Work out the finished part from the listing and answer in its coordinate system (mm). Round coordinates to 2 decimals unless told otherwise and drop trailing zeros. Order: outer loops, then holes, each group sorted by start corner. A loop starts at its lowest first (then second) coordinate and runs counter-clockwise, first axis right, second up. Notation, with made-up numbers: M 15,63 L 69,63 A14 ccw 69,79 Z; hole C 66,21 d8. An arc over 180 degrees is marked long. Answer as a JSON object with one key per item and string values. Group by question number.
Autodesk Inventor part; units mm, degrees
ref_plane "YZ Plane" through (0, 0, 0) normal (1, 0, 0) x (0, 1, 0)
ref_plane "XZ Plane" through (0, 0, 0) normal (0, 1, 0) x (-1, 0, 0)
ref_plane "XY Plane" through (0, 0, 0) normal (0, 0, 1) x (1, 0, 0)
sketch "Skizze1" plane through (0, 0, 0) normal (0, 0, 1) x (1, 0, 0)
  line L0 (0, 0) -> (12.8, 0)
  line L1 (12.8, 0) -> (12.8, 6.5)
  line L2 (12.8, 6.5) -> (0, 6.5)
  line L3 (0, 6.5) -> (0, 0)
  circle A0 centre (3.15, 1.5) radius 0.7
  circle A1 centre (9.65, 1.5) radius 0.7
  line L4 (3.15, 1.5) -> (9.65, 1.5) construction
  line L5 (6.4, 0) -> (6.4, 6.5) construction
  dimension "d0" = 12.8
  dimension "d1" = 6.5
  dimension "d2" = 1.5
  dimension "d3" = 3.15
  dimension "d4" = 6.5
  dimension "d7" = 1.4
extrude "Extrusion1" add sketch "Skizze1" along normal blind 5.8
ref_plane "Arbeitsebene1" through (0, 0, 2.9) normal (0, 0, 1) x (1, 0, 0)
sketch "Skizze2" plane through (0, 0, 2.9) normal (0, 0, 1) x (1, 0, 0)
  circle A0 centre (3.15, 1.5) radius 0.7 construction
  line L0 (0, 0) -> (12.8, 0)
  line L1 (13.95, 8.3) -> (1, 6.5)
  line L2 (12.8, 6.5) -> (0, 6.5)
  line L3 (13.95, 11.5) -> (1, 6.5) construction
  line L4 (0, 6.5) -> (0, 0)
  line L5 (13.95, 8.3) -> (14.0188, 7.8048)
  line L6 (14.0188, 7.8048) -> (1.0688, 6.0048)
  line L7 (1.0688, 6.0048) -> (1, 6.5)
  point P0 (4.6318, 6.5)
  dimension "d8" = 10.8
  dimension "d9" = 10.8
  dimension "d10" = 8.3
  dimension "d11" = 11.5
  dimension "d12" = 1
  dimension "d13" = 0.5
equation "\"d9\" = d8"
properties part number "LimitSwitch"
Item 1: The mould has two halves that part along X. Classify faces 1 (the flat face through (6, 3, 0)), 2 (the flat face through (0, 3, 3)), 3 (the cylindrical face through (2.595, 1.926, 2.859)), 4 (the cylindrical face through (8.95, 1.47, 2.86)): +X half, -X half, draft (parallel to the pull), parting line (faces both ways), or undercut.
Item 2: Find section A-A (x = 3.15). Give the vertices of the cut face in (y, z).
Item 3: Find section C-C (z = 2.65). Give the vertices of the cut face in (x, y).
Item 4: Find section B-B (y = 1.5). Give the vertices of the cut face in (x, z).
Item 5: Consider L1, parallel to Y at x = 3.15, z = 4.3; L2, parallel to X at y = 1, z = 3.4; L3, parallel to Y at x = 9.25, z = 2.5. Determine where each line is inside the solid, lowest interval first.
Responses:
{
 "1": {"face 1": "draft", "face 2": "-X half", "face 3": "undercut", "face 4": "undercut"},
 "2": {"outline": "M 0,0 L 0.8,0 L 0.8,5.8 L 0,5.8 Z; M 2.2,0 L 6.5,0 L 6.5,5.8 L 2.2,5.8 Z"},
 "3": {"outline": "M 0,0 L 12.8,0 L 12.8,6.5 L 0,6.5 Z; hole C 3.15,1.5 d1.4; hole C 9.65,1.5 d1.4"},
 "4": {"outline": "M 0,0 L 2.45,0 L 2.45,5.8 L 0,5.8 Z; M 3.85,0 L 8.95,0 L 8.95,5.8 L 3.85,5.8 Z; M 10.35,0 L 12.8,0 L 12.8,5.8 L 10.35,5.8 Z"},
 "5": {"L1": "y = 0 to 0.8, 2.2 to 6.5", "L2": "x = 0 to 2.66, 3.64 to 9.16, 10.14 to 12.8", "L3": "y = 0 to 0.93, 2.07 to 6.5"}
}
